from build123d import *

# Parameters (mm, degrees)
SKETCH1_R           = 3.1496
BOSS_EXTRUDE1_DEPTH = 3.175


with BuildPart() as part:
    # Sketch1 → Boss-Extrude1 (new body)
    with BuildSketch(Plane.XY):
        with BuildLine():
            Line((0.762, 0), (103.378, 0))
            ThreePointArc((103.378, 0), (103.916815367, 0.223184633), (104.14, 0.762))
            Line((104.14, 0.762), (104.14, 5.08))
            Line((104.14, 5.08), (117.348, 5.08))
            ThreePointArc((117.348, 5.08), (117.886815367, 5.303184633), (118.11, 5.842))
            Line((118.11, 5.842), (118.11, 10.668))
            ThreePointArc((118.11, 10.668), (117.886815367, 11.206815367), (117.348, 11.43))
            Line((117.348, 11.43), (104.14, 11.43))
            Line((104.14, 11.43), (104.14, 24.638))
            ThreePointArc((104.14, 24.638), (103.916815367, 25.176815367), (103.378, 25.4))
            Line((103.378, 25.4), (0.762, 25.4))
            ThreePointArc((0.762, 25.4), (0.223184633, 25.176815367), (0, 24.638))
            Line((0, 24.638), (0, 11.43))
            Line((0, 11.43), (-13.208, 11.43))
            ThreePointArc((-13.208, 11.43), (-13.746815367, 11.206815367), (-13.97, 10.668))
            Line((-13.97, 10.668), (-13.97, 5.842))
            ThreePointArc((-13.97, 5.842), (-13.746815367, 5.303184633), (-13.208, 5.08))
            Line((-13.208, 5.08), (0, 5.08))
            Line((0, 5.08), (0, 0.762))
            ThreePointArc((0, 0.762), (0.223184633, 0.223184633), (0.762, 0))
        make_face()
        with Locations((52.07, 12.7)):
            Circle(SKETCH1_R, mode=Mode.SUBTRACT)
    extrude(amount=BOSS_EXTRUDE1_DEPTH)


solid = part.part
Read the model definition and answer for the solid it produces. Units are mm, in the model's axes. A direction names the side the tool comes from. Give positions to 0.01 mm unless a question says otherwise; leave off trailing zeros. Loops run counter-clockwise (first coordinate to the right, second up) from the corner with the lowest first, then second, coordinate; pieces in that order, holes last. Notation, with made-up numbers: M 75.5,17.5 L 130.5,17.5 A18 cw 130.5,24.5 Z; hole C 30.25,41.25 d11. An arc over 180 degrees is marked long. Write each question's results on one line, items separated by ' | '.
1. Section B-B on x = 52.07 is taken. Give the vertices of the cut face in (y, z) (3 decimals), plus the area to 3 significant figures.
Values:
outline: M 0,0 L 9.55,0 L 9.55,3.175 L 0,3.175 Z; M 15.85,0 L 25.4,0 L 25.4,3.175 L 15.85,3.175 Z | area: 60.6 mm^2
2. A tool of negligible diameter and unlimited length cuts with its end or side. For faces 4 (the face through (0, 18, 2)), 5 (the face through (51, 0, 2)), 6 (the face through (104.14, 18, 2)), 7 (the face through (104.14, 3, 2)), 8 (the face through (-13.97, 8, 2)), from which of +Z, -Z, +X, -X, +Y, -Y can it reach the whole face along a straight path? Write none if from no direction.
Values:
face 4: +Z, -Z, -X, +Y | face 5: +Z, -Z, +X, -X, -Y | face 6: +Z, -Z, +X, +Y | face 7: +Z, -Z, +X, -Y | face 8: +Z, -Z, -X, +Y, -Y
3. Section D-D on y = 17.5 is taken. Give the vertices of the cut face in (x, z) (3 decimals), plus the area to 3 significant figures.
Values:
outline: M 0,0 L 104.14,0 L 104.14,3.175 L 0,3.175 Z | area: 331 mm^2
4. Straight lines are drawn through the part: line 1 (Y direction, x = 52.07, z = 1.15); line 2 (X direction, y = 1.75, z = 2.2); line 3 (X direction, y = 15, z = 1). For each, find the intervals that lie inside material, in ascending order. Write a range as [from, to].
Values:
line 1: y = [0, 9.55], [15.85, 25.4] | line 2: x = [0, 104.14] | line 3: x = [0, 49.92], [54.22, 104.14]
5. Section A-A on z = 2.4 is taken. Give the vertices of the cut face in (x, y), plus the area to 3 significant figures.
Values:
outline: M -13.97,5.84 A0.76 ccw -13.21,5.08 L 0,5.08 L 0,0.76 A0.76 ccw 0.76,0 L 103.38,0 A0.76 ccw 104.14,0.76 L 104.14,5.08 L 117.35,5.08 A0.76 ccw 118.11,5.84 L 118.11,10.67 A0.76 ccw 117.35,11.43 L 104.14,11.43 L 104.14,24.64 A0.76 ccw 103.38,25.4 L 0.76,25.4 A0.76 ccw 0,24.64 L 0,11.43 L -13.21,11.43 A0.76 ccw -13.97,10.67 Z; hole C 52.07,12.7 d6.3 | area: 2,790 mm^2
6. The mould has two halves that part along Y. Classify faces 1 (the face through (-7, 5.08, 2)), 2 (the face through (54.98, 11.49, 1.57)), 3 (the face through (0, 3, 2)): pulls with the +Y half, pulls with the -Y half, needs draft (parallel to the pull), parting line crosses it, or undercut.
Values:
face 1: pulls with the -Y half | face 2: undercut | face 3: needs draft
7. Section C-C on y = 12.7 is taken. Give the vertices of the cut face in (x, z) (3 decimals), plus the area to 3 significant figures.
Values:
outline: M 0,0 L 48.92,0 L 48.92,3.175 L 0,3.175 Z; M 55.22,0 L 104.14,0 L 104.14,3.175 L 55.22,3.175 Z | area: 311 mm^2
8. Given pin 1 (1.6 mm diameter, centred on y = 4, z = 1, fed in from +X); pin 2 (1.6 mm diameter, centred on x = -7, z = 2, fed in from +Y); pin 3 (1 mm diameter, centred on y = 15.5, z = 1.5, fed in from -X); pin 4 (5.5 mm diameter, centred on x = 52.07, y = 12.7, fed in from -Z), each flat-ended and moving along its own axis, determine where each tip first touches the part or whether it passes through.
Values:
pin 1: stops at x = 104.14 | pin 2: stops at y = 11.43 | pin 3: stops at x = 0 | pin 4: passes through
